from build123d import *

# Parameters (mm, degrees)
BOSS_EXTRUDE1_DEPTH = 88
FILLET1_R           = 1


with BuildPart() as part:
    # Sketch1 → Boss-Extrude1 (new body)
    with BuildSketch(Plane.XY):
        with BuildLine():
            Line((-175, -3.5), (175, -3.5))
            ThreePointArc((175, -3.5), (248.475712044, 71.889375453), (171.222497777, 143.402864229))
            Line((171.222497777, 143.402864229), (-178.31495093, 125.414758405))
            ThreePointArc((-178.31495093, 125.414758405), (-239.47868608, 59.341976644), (-175, -3.5))
        make_face()
        with BuildLine():
            Line((-175, 0), (175, 0))
            ThreePointArc((175, 0), (244.976868614, 71.799405193), (171.402378835, 139.907489741))
            Line((171.402378835, 139.907489741), (-178.135069872, 121.919383918))
            ThreePointArc((-178.135069872, 121.919383918), (-235.979842649, 59.431946903), (-175, 0))
        make_face(mode=Mode.SUBTRACT)
    extrude(amount=BOSS_EXTRUDE1_DEPTH)

    # Fillet1
    fillet1_edges = [part.edges().sort_by_distance(p)[0] for p in [
        (248.475712044, 71.889375453, 88),
        (-235.979842649, 59.431946903, 0),
        (0, 0, 0),
        (244.976868614, 71.799405193, 0),
        (-3.366345518, 130.91343683, 0),
        (-235.979842649, 59.431946903, 88),
        (-3.546226577, 134.408811317, 88),
        (0, 0, 88),
        (244.976868614, 71.799405193, 88),
        (-3.366345518, 130.91343683, 88),
        (-239.47868608, 59.341976644, 88),
        (-3.546226577, 134.408811317, 0),
        (248.475712044, 71.889375453, 0),
        (0, -3.5, 0),
        (-239.47868608, 59.341976644, 0),
        (0, -3.5, 88),
    ]]
    fillet(fillet1_edges, radius=FILLET1_R)


solid = part.part
Build history of the part. All positions in model axes, mm. A direction names the side the tool comes from. Give positions to 0.01 mm unless a question says otherwise; leave off trailing zeros. Write each loop counter-clockwise with the first axis right and the second up, starting at its lowest first coordinate (ties: lowest second). Pieces come first, ordered by that corner, then holes. Notation, with made-up numbers: (-31.75, 1) - (10.25, 1) arc R17 cw to (10.25, 33) - close; hole circle Ø9 at (-19, -2.5). An arc over 180 degrees is marked (long way). Use one line per item in the form item = value. Start each with the question number.
1. Drop flat-ended pins along their axis: pin 1 Ø3 at (x, z) = (16.5, 74) entering from +Y; pin 2 Ø5 at (y, z) = (119, 66.5) entering from +X; pin 3 Ø4 at (x, z) = (-93.5, 40) entering from +Y. Give the stop position or say it passes through.
2. Probe line 1 (X direction, y = 45, z = 78.5); line 2 (X direction, y = 15.5, z = 36); line 3 (Y direction, x = -9, z = 47). List the from-to ranges inside material, lowest first. Write a range as [from, to].
3. Band-saw the part on A-A on z = 24. Write the cut outline in (x, y), plus the area to 3 significant figures.
4. Two-plate mould, pull along X, no slides. Class faces 1 (the face through (-2, 0, 43)), 2 (the face through (245, 70, 43)), 3 (the face through (-2, -3.5, 43)), 4 (the face through (-239.5, 60.7, 43.4)): released by +X, released by -X, zero draft, split by the parting line, or undercut.
5. 3-axis set-ups, long thin cutter, end or side, ignore diameter. For faces 5 (the face through (-5.828, 131.072, 87.699)), 6 (the face through (-0.92, 131.04, 43.4)), 7 (the face through (-5.98, 134, 87.7)), 8 (the face through (-5.828, 131.072, 0.301)): which of +Z, -Z, +X, -X, +Y, -Y reach the whole face in a straight line?
Conclusion:
q1.pin_1 = 135.52
q1.pin_2 = 231.92
q1.pin_3 = 129.88
q2.line_1 = [-237.48, -233.86], [240.38, 244.12]
q2.line_2 = [-220.72, -215.63], [218.93, 224.32]
q2.line_3 = [-3.5, 0], [130.62, 134.13]
q3.outline = (-178.31, 125.41) arc R64.5 ccw to (-175, -3.5) - (175, -3.5) arc R73.5 ccw (long way) to (171.22, 143.4) - close; hole (-178.14, 121.92) arc R61 ccw to (-175, 0) - (175, 0) arc R70 ccw (long way) to (171.4, 139.91) - close
q3.area = 3,930 mm²
q4.face_1 = undercut
q4.face_2 = undercut
q4.face_3 = zero draft
q4.face_4 = released by -X
q5.face_5 = +Z
q5.face_6 = +Z, -Z
q5.face_7 = +Z, -X, +Y
q5.face_8 = -Z
